from build123d import *

# Parameters (mm, degrees)
SKETCH1_R          = 6.1
BASEHEAD_DEPTH     = 8
SKETCH2_OUTSIDE_W  = 18.004
SKETCH2_OUTSIDE_H  = 18.004
CUT_EXTRUDE1_DEPTH = 8
FILLET1_R          = 0.8


with BuildPart() as part:
    # Sketch1 → BaseHead (new body)
    with BuildSketch(Plane(origin=(0, 0, 0), x_dir=(0, 0, -1), z_dir=(1, 0, 0))):
        Circle(SKETCH1_R)
    extrude(amount=BASEHEAD_DEPTH)

    # Sketch2 outside → Cut-Extrude1 (cut)
    with BuildSketch(Plane(origin=(0, 2.662946325, -1.492108674), x_dir=(0, 0, 1), z_dir=(-1, 0, 0))):
        with Locations((1.492, -2.663)):
            Rectangle(SKETCH2_OUTSIDE_W, SKETCH2_OUTSIDE_H)
        Polygon((8.563176486, -2.662946325), (1.492108674, 4.408121487), (-5.578959138, -2.662946325), (1.492108674, -9.734014137), align=None, mode=Mode.SUBTRACT)
    extrude(amount=-CUT_EXTRUDE1_DEPTH, mode=Mode.SUBTRACT)

    # Sketch3 → Cut-Revolve1 (revolve, cut)
    with BuildSketch(Plane(origin=(1.259716749, -5.274716749, 0), x_dir=(0, -1, 0), z_dir=(0, 0, 1))):
        Polygon((-11.984716749, -1.259716749), (-10.274716749, -1.259716749), (-11.984716749, -0.272447788), align=None)
    revolve(axis=Axis((1.545283251, 0, 0), (-1, 0, 0)), mode=Mode.SUBTRACT)

    # Sketch4 → BaseBody (revolve)
    with BuildSketch(Plane(origin=(-10.34721472, 12.84721472, 0), x_dir=(0, -1, 0), z_dir=(0, 0, 1)), mode=Mode.PRIVATE) as basebody_sk:
        Polygon((12.84721472, 18.34721472), (17.84721472, 18.34721472), (17.84721472, 52.04721472), (16.34721472, 52.04721472), (16.34721472, 54.84721472), (12.84721472, 58.34721472), align=None)
    revolve(basebody_sk.sketch.rotate(Axis((14.086803097, 0, 0), (-1, 0, 0)), 180), axis=Axis((14.086803097, 0, 0), (-1, 0, 0)))

    # Fillet1
    fillet1_edges = [part.edges().sort_by_distance(p)[0] for p in [
        (41.7, -3.5, 0),
    ]]
    fillet(fillet1_edges, radius=FILLET1_R)


solid = part.part
The listing builds one solid part. Answer for the finished solid, in the listing's coordinates (mm). A direction names the side the tool comes from. Coordinates: 2 decimals unless noted, no trailing zeros. Write each loop counter-clockwise with the first axis right and the second up, starting at its lowest first coordinate (ties: lowest second). Pieces come first, ordered by that corner, then holes. Notation, with made-up numbers: M -18,-7 L -8,-7 A28 cw -8,19 Z; hole C 63.25,20 d7. An arc over 180 degrees is marked long. Put each result on its own line as item: value. Start each with the question number.
1. A cutting plane is placed at A-A on x = 22. Write down the section's boundary in (y, z), then the cut area to 3 significant figures.
2. Consider line 1 (Y direction, x = 39, z = 0.25); line 2 (X direction, y = 4, z = 2); line 3 (Z direction, x = 20, y = 2.25). Determine where each line is inside the solid, lowest interval first. Write a range as from..to.
3. Flat-ended cylindrical pins translate along their axes: P1, Ø1.3, axis at y = -5.5, z = -1.5, coming from the +X side; P2, Ø2, axis at y = -1, z = 5.5, coming from the +X side; P3, Ø1.5, axis at x = 34, y = 3, coming from the -Z side. Find the tip coordinate at first contact, or state that the pin passes through.
4. A cutting plane is placed at B-B on x = 44. Write down the section's boundary in (y, z), then the cut area to 3 significant figures.
5. Which of the six approach directions +Z, -Z, +X, -X, +Y, -Y give full straight-line access (tool end or side, diameter ignored) to faces 1 (the cylindrical face through (25, -5, 0)), 2 (the conical face through (0.18, -5.31, -0.06))?
Resolved:
1. outline: C 0,0 d10
1. area: 78.5 mm2
2. line 1: y = -4.99..4.99
2. line 2: x = 0..41.7
2. line 3: z = -4.47..4.47
3. P1: stops at x = 8
3. P2: stops at x = 41.7
3. P3: stops at z = -4.47
4. outline: C 0,0 d7
4. area: 38.5 mm2
5. face 1: +X
5. face 2: -X, -Y
